```python
from build123d import *

# Parameters (mm, degrees)
SKETCH2_W           = 90
SKETCH2_H           = 40
BOSS_EXTRUDE1_DEPTH = 5
CUT_EXTRUDE1_DEPTH  = 10


with BuildPart() as part:
    # Sketch2 → Boss-Extrude1 (new body)
    with BuildSketch(Plane(origin=(0, 0, 0), x_dir=(-1, 0, 0), z_dir=(0, 1, 0))):
        Polygon((-50, -12.990381057), (-50, 12.990381057), (-27.5, 0), align=None)
        Rectangle(SKETCH2_W, SKETCH2_H)
        Polygon((50, 12.990381057), (27.5, 0), (50, -12.990381057), align=None)
        Polygon((12.990381057, 25), (-12.990381057, 25), (0, 2.5), align=None)
        Polygon((0, -2.5), (12.990381057, -25), (-12.990381057, -25), align=None)
    extrude(amount=BOSS_EXTRUDE1_DEPTH)

    # Sketch3 → Cut-Extrude1 (cut)
    with BuildSketch(Plane(origin=(0, 5, 0), x_dir=(-1, 0, 0), z_dir=(0, 1, 0))):
        Polygon((-16.3, -7.529573217), (-16.3, -15), (21.7, -15), (21.7, -5), (-16.3, -5), align=None)
    extrude(amount=-CUT_EXTRUDE1_DEPTH, mode=Mode.SUBTRACT)


solid = part.part
```
CAD build for the part. Positions are in the model's coordinates, mm. A direction names the side the tool comes from. Round coordinates to 2 decimals unless told otherwise and drop trailing zeros. Loops run counter-clockwise (first coordinate to the right, second up) from the corner with the lowest first, then second, coordinate; pieces in that order, holes last. Notation, with made-up numbers: (33, 76.5) - (91, 76.5) arc R21 cw to (91, 108.5) - close; hole circle Ø9 at (74.5, -5). An arc over 180 degrees is marked (long way). Return JSON: item names as keys, results as strings. Group by question number.
Q1. Band-saw the part on B-B on x = -5. Give the cut face in (y, z).
Q2. Band-saw the part on A-A on z = -8.5. Give the cut face in (x, y), plus the area to 3 significant figures.
Q3. Two-plate mould, pull along X, no slides. Class faces 1 (the face through (-21.7, 3, -10)), 2 (the face through (-50, 2, 0)), 3 (the face through (28, 2, -20)), 4 (the face through (50, 2, 0)): +X half, -X half, draft (parallel to the pull), parting line (faces both ways), or undercut.
Q4. Band-saw the part on D-D on z = 12. Give the cut face in (x, y), plus the area to 3 significant figures.
Q5. Drill centre lines: line 1 along Z through (x, y) = (0, 1.5); line 2 along Z through (x, y) = (12, 0.3); line 3 along X through (y, z) = (2.6, -9.5). Where is each one in solid material? Low to high. Write a range as [from, to].
Q6. Flat gauge pins, fed straight in: pin 1 Ø1.5 at (y, z) = (2.5, -16) entering from +X; pin 2 Ø2.5 at (x, y) = (-20.5, 2.5) entering from -Z; pin 3 Ø1.5 at (y, z) = (3, -16) entering from -X. Where does each tip first touch, or does it go through?
Q7. Band-saw the part on C-C on y = 3.9. Give the cut face in (x, z), plus the area to 3 significant figures.
Q8. Tool access for faces 5 (the face through (47.54, 2.46, 11.57)), 6 (the face through (-11.527, 2.465, -22.465)), 7 (the face through (-3, 3, -5)), 8 (the face through (11.57, 2.46, 22.54)), 9 (the face through (-47.465, 2.465, -11.527)): list every direction of +Z, -Z, +X, -X, +Y, -Y with a clear straight run to the whole face (end or side of a thin tool).
Solutions:
{
 "1": {"outline": "(0, -25) - (5, -25) - (5, -15) - (0, -15) - close; (0, -5) - (5, -5) - (5, 25) - (0, 25) - close"},
 "2": {"outline": "(-50, 0) - (-21.7, 0) - (-21.7, 5) - (-50, 5) - close; (16.3, 0) - (50, 0) - (50, 5) - (16.3, 5) - close", "area": "310 mm^2"},
 "3": {"face 1": "undercut", "face 2": "-X half", "face 3": "draft", "face 4": "+X half"},
 "4": {"outline": "(-50, 0) - (-48.28, 0) - (-48.28, 5) - (-50, 5) - close; (-45, 0) - (45, 0) - (45, 5) - (-45, 5) - close; (48.28, 0) - (50, 0) - (50, 5) - (48.28, 5) - close", "area": "467 mm^2"},
 "5": {"line 1": "z = [-25, -15], [-5, 25]", "line 2": "z = [-25, -23.28], [-20, -15], [-5, 20], [23.28, 25]", "line 3": "x = [-50, -21.7], [16.3, 50]"},
 "6": {"pin 1": "stops at x = 45", "pin 2": "stops at z = -20", "pin 3": "stops at x = -45"},
 "7": {"outline": "(-50, -12.99) - (-45, -10.1) - (-45, -20) - (-10.1, -20) - (-12.99, -25) - (12.99, -25) - (10.1, -20) - (45, -20) - (45, -10.1) - (50, -12.99) - (50, 12.99) - (45, 10.1) - (45, 20) - (10.1, 20) - (12.99, 25) - (-12.99, 25) - (-10.1, 20) - (-45, 20) - (-45, 10.1) - (-50, 12.99) - close; hole (-21.7, -15) - (16.3, -15) - (16.3, -5) - (-21.7, -5) - close", "area": "3,680 mm^2"},
 "8": {"face 5": "+Z, +Y, -Y", "face 6": "-X, +Y, -Y", "face 7": "+Y, -Y", "face 8": "+X, +Y, -Y", "face 9": "-Z, +Y, -Y"}
}
